Geometry check sheet. Reference: the model listing, model coordinates, mm. Give positions to 0.01 mm unless a question says otherwise; leave off trailing zeros. Loops run counter-clockwise (first coordinate to the right, second up) from the corner with the lowest first, then second, coordinate; pieces in that order, holes last. Notation, with made-up numbers: (-25, 58) - (22, 58) arc R16 ccw to (22, 74) - close; hole circle Ø7 at (13.25, 11). An arc over 180 degrees is marked (long way). Use a Markdown table: item, result. Add a question column.
1. Material ranges on L1, parallel to Y at x = 285, z = 0 (1 decimal); L2, parallel to Y at x = -336, z = 1, recorded low to high.
2. Cross-section at A-A on z = 0. Enter the section's corners in (x, y) (1 decimal), and give its area (3 significant figures).
3. Depth check by flat-ended pin: P1, Ø5, axis at x = 352, z = 4, coming from the -Y side; P2, Ø3, axis at x = 351.5, z = -2.5, coming from the -Y side; P3, Ø8, axis at x = -128, y = -4.5, coming from the +Z side. Enter the tip coordinate at first touch or a pass-through.
from build123d import *

# Parameters (mm, degrees)
SKETCH_1_R        = 7.9375
SKETCH_1_R_2      = 3.975
EXTRUDE_1_DEPTH   = 614.3625
FILLET_1_R        = 2.5
MOVE_BODY_1_ANGLE = 90


with BuildPart() as part:
    # 스케치1 → 보스-돌출1 (new body, symmetric)
    with BuildSketch(Plane(origin=(0, 0, 0), x_dir=(1, 0, 0), z_dir=(0, 1, 0))):
        Circle(SKETCH_1_R)
        Circle(SKETCH_1_R_2, mode=Mode.SUBTRACT)
    extrude(amount=EXTRUDE_1_DEPTH, both=True)

    # 필렛1
    fillet_1_edges = [part.edges().sort_by_distance(p)[0] for p in [
        (-7.9375, -614.3625, 0),
        (-7.9375, 614.3625, 0),
    ]]
    fillet(fillet_1_edges, radius=FILLET_1_R)


with BuildPart() as part_1:
    # Move Body 1: moved
    add(part.part.rotate(Axis((0, 0, 0), (0, 0, 1)), MOVE_BODY_1_ANGLE))


solid = part_1.part
Values found:
| question | item | result |
|---|---|---|
| 1 | L1 | y = -7.9 to -4, 4 to 7.9 |
| 1 | L2 | y = -7.87 to -3.85, 3.85 to 7.87 |
| 2 | outline | (-614.4, -5.4) arc R2.5 ccw to (-611.9, -7.9) - (611.9, -7.9) arc R2.5 ccw to (614.4, -5.4) - (614.4, -4) - (-614.4, -4) - close; (-614.4, 4) - (614.4, 4) - (614.4, 5.4) arc R2.5 ccw to (611.9, 7.9) - (-611.9, 7.9) arc R2.5 ccw to (-614.4, 5.4) - close |
| 2 | area | 9,730 mm2 |
| 3 | P1 | stops at y = -7.79 |
| 3 | P2 | stops at y = -7.87 |
| 3 | P3 | stops at z = 7.92 |
